from build123d import *

# Parameters (mm, degrees)
F1_DEPTH = 2.921
F2_R     = 1.65
F3_DEPTH = 25.4
F4_W     = 8.591786
F4_H     = 32.204256
F5_DEPTH = 25.4
F6_R     = 0.254


with BuildPart() as f1:
    # F0 (on Front) → F1 (new body, symmetric)
    with BuildSketch(Plane.XZ):
        with BuildLine():
            Line((4.445, -12.7), (4.445, 12.7))
            Line((4.445, 12.7), (-4.445, 12.7))
            ThreePointArc((-4.445, 12.7), (-3.7846, 12.0396), (-4.445, 11.3792))
            Line((-4.445, 11.3792), (-4.445, 10.6934))
            ThreePointArc((-4.445, 10.6934), (-3.7846, 10.033), (-4.445, 9.3726))
            Line((-4.445, 9.3726), (-4.445, 8.6868))
            ThreePointArc((-4.445, 8.6868), (-3.7846, 8.0264), (-4.445, 7.366))
            Line((-4.445, 7.366), (-4.445, 6.6802))
            ThreePointArc((-4.445, 6.6802), (-3.7846, 6.0198), (-4.445, 5.3594))
            Line((-4.445, 5.3594), (-4.445, 4.6736))
            ThreePointArc((-4.445, 4.6736), (-3.7846, 4.0132), (-4.445, 3.3528))
            Line((-4.445, 3.3528), (-4.445, 2.667))
            ThreePointArc((-4.445, 2.667), (-3.7846, 2.0066), (-4.445, 1.3462))
            Line((-4.445, 1.3462), (-4.445, 0.6604))
            ThreePointArc((-4.445, 0.6604), (-3.7846, 0), (-4.445, -0.6604))
            Line((-4.445, -0.6604), (-4.445, -1.3462))
            ThreePointArc((-4.445, -1.3462), (-3.7846, -2.0066), (-4.445, -2.667))
            Line((-4.445, -2.667), (-4.445, -3.3528))
            ThreePointArc((-4.445, -3.3528), (-3.7846, -4.0132), (-4.445, -4.6736))
            Line((-4.445, -4.6736), (-4.445, -5.3594))
            ThreePointArc((-4.445, -5.3594), (-3.7846, -6.0198), (-4.445, -6.6802))
            Line((-4.445, -6.6802), (-4.445, -7.366))
            ThreePointArc((-4.445, -7.366), (-3.7846, -8.0264), (-4.445, -8.6868))
            Line((-4.445, -8.6868), (-4.445, -9.3726))
            ThreePointArc((-4.445, -9.3726), (-3.7846, -10.033), (-4.445, -10.6934))
            Line((-4.445, -10.6934), (-4.445, -11.3792))
            ThreePointArc((-4.445, -11.3792), (-3.7846, -12.0396), (-4.445, -12.7))
            Line((-4.445, -12.7), (4.445, -12.7))
        make_face()
        with BuildLine():
            ThreePointArc((-4.445, 11.3792), (-3.7846, 12.0396), (-4.445, 12.7))
            Line((-4.445, 12.7), (-4.445, 11.3792))
        make_face()
        with BuildLine():
            Line((-4.445, -11.5316), (-4.445, -12.7))
            ThreePointArc((-4.445, -12.7), (-3.7846, -12.0396), (-4.445, -11.3792))
            Line((-4.445, -11.3792), (-4.445, -11.5316))
        make_face()
        with BuildLine():
            ThreePointArc((-4.445, 9.3726), (-3.7846, 10.033), (-4.445, 10.6934))
            Line((-4.445, 10.6934), (-4.445, 10.541))
            Line((-4.445, 10.541), (-4.445, 9.3726))
        make_face()
        with BuildLine():
            Line((-4.445, -9.525), (-4.445, -10.6934))
            ThreePointArc((-4.445, -10.6934), (-3.7846, -10.033), (-4.445, -9.3726))
            Line((-4.445, -9.3726), (-4.445, -9.525))
        make_face()
        with BuildLine():
            ThreePointArc((-4.445, 7.366), (-3.7846, 8.0264), (-4.445, 8.6868))
            Line((-4.445, 8.6868), (-4.445, 8.5344))
            Line((-4.445, 8.5344), (-4.445, 7.366))
        make_face()
        with BuildLine():
            Line((-4.445, -7.5184), (-4.445, -8.6868))
            ThreePointArc((-4.445, -8.6868), (-3.7846, -8.0264), (-4.445, -7.366))
            Line((-4.445, -7.366), (-4.445, -7.5184))
        make_face()
        with BuildLine():
            ThreePointArc((-4.445, 5.3594), (-3.7846, 6.0198), (-4.445, 6.6802))
            Line((-4.445, 6.6802), (-4.445, 6.5278))
            Line((-4.445, 6.5278), (-4.445, 5.3594))
        make_face()
        with BuildLine():
            Line((-4.445, -5.5118), (-4.445, -6.6802))
            ThreePointArc((-4.445, -6.6802), (-3.7846, -6.0198), (-4.445, -5.3594))
            Line((-4.445, -5.3594), (-4.445, -5.5118))
        make_face()
        with BuildLine():
            ThreePointArc((-4.445, 3.3528), (-3.7846, 4.0132), (-4.445, 4.6736))
            Line((-4.445, 4.6736), (-4.445, 4.5212))
            Line((-4.445, 4.5212), (-4.445, 3.3528))
        make_face()
        with BuildLine():
            Line((-4.445, -3.5052), (-4.445, -4.6736))
            ThreePointArc((-4.445, -4.6736), (-3.7846, -4.0132), (-4.445, -3.3528))
            Line((-4.445, -3.3528), (-4.445, -3.5052))
        make_face()
        with BuildLine():
            ThreePointArc((-4.445, 1.3462), (-3.7846, 2.0066), (-4.445, 2.667))
            Line((-4.445, 2.667), (-4.445, 2.5146))
            Line((-4.445, 2.5146), (-4.445, 1.3462))
        make_face()
        with BuildLine():
            Line((-4.445, -1.4986), (-4.445, -2.667))
            ThreePointArc((-4.445, -2.667), (-3.7846, -2.0066), (-4.445, -1.3462))
            Line((-4.445, -1.3462), (-4.445, -1.4986))
        make_face()
        with BuildLine():
            ThreePointArc((-4.445, -0.6604), (-3.7846, 0), (-4.445, 0.6604))
            Line((-4.445, 0.6604), (-4.445, 0.508))
            Line((-4.445, 0.508), (-4.445, -0.6604))
        make_face()
    extrude(amount=F1_DEPTH, both=True)

    # F2 (on face) → F3 (cut)
    with BuildSketch(Plane.YZ.offset(4.445)):
        Circle(F2_R)
    extrude(amount=-F3_DEPTH, mode=Mode.SUBTRACT)

    # F4 (on face) → F5 (cut)
    with BuildSketch(Plane(origin=(0, 2.921, 0), x_dir=(-1, 0, 0), z_dir=(0, 1, 0))):
        with Locations((-6.200893, 0)):
            Rectangle(F4_W, F4_H)
    extrude(amount=-F5_DEPTH, mode=Mode.SUBTRACT)

    # F6
    f6_edges = [f1.edges().sort_by_distance(p)[0] for p in [
        (-4.445, 0, 12.7),
        (-4.445, 0, -12.7),
    ]]
    fillet(f6_edges, radius=F6_R)


solid = f1.part
CAD build for the part. Positions are in the model's coordinates, mm. Round coordinates to 2 decimals unless told otherwise and drop trailing zeros. Order: outer loops, then holes, each group sorted by start corner. A loop starts at its lowest first (then second) coordinate and runs counter-clockwise, first axis right, second up. Notation, with made-up numbers: (44, -9) - (83, -9) arc R28 cw to (83, 15) - close; hole circle Ø11 at (19.25, 86). An arc over 180 degrees is marked (long way). Return JSON: item names as keys, results as strings.
(1) Cut at C-C (x = 1.25). Give the cut face in (y, z), then the cut area to 3 significant figures.
Answer key:
{"outline": "(-2.92, -12.7) - (2.92, -12.7) - (2.92, 12.7) - (-2.92, 12.7) - close; hole circle Ø3.3 at (0, 0)", "area": "140 mm^2"}
(2) Wall check: probe 1 along Z at (x, y) = (-1, 0); probe 2 along Y at (x, z) = (0.5, 1). Give the ranges that are in metal, low to high. Write a range as from..to.
Answer key:
{"probe 1": "z = -12.7..-1.65, 1.65..12.7", "probe 2": "y = -2.92..-1.31, 1.31..2.92"}
(3) Pull direction Z, two halves, no side cores. Call faces 1 (the face through (-1.226, -1.216, 1.115)), 2 (the face through (-1, 2.921, 0)), 3 (the face through (-1, 0, -12.7)), 4 (the face through (-1, 0, 12.7)): +Z half, -Z half, draft (parallel to the pull), parting line (faces both ways), or undercut.
Answer key:
{"face 1": "undercut", "face 2": "draft", "face 3": "-Z half", "face 4": "+Z half"}
(4) Cut at B-B (y = 0). Give the cut face in (x, z) (3 decimals).
Answer key:
{"outline": "(-4.445, -12.446) arc R0.254 ccw to (-4.191, -12.7) - (1.905, -12.7) - (1.905, -1.65) - (-4.445, -1.65) - close; (-4.445, 1.65) - (1.905, 1.65) - (1.905, 12.7) - (-4.191, 12.7) arc R0.254 ccw to (-4.445, 12.446) - close"}
(5) Cut at A-A (z = 0). Give the cut face in (x, y) (3 decimals), then the cut area to 3 significant figures.
Answer key:
{"outline": "(-4.445, -2.921) - (1.905, -2.921) - (1.905, -1.65) - (-4.445, -1.65) - close; (-4.445, 1.65) - (1.905, 1.65) - (1.905, 2.921) - (-4.445, 2.921) - close", "area": "16.1 mm^2"}
